from build123d import *

# Parameters (mm, degrees)
SKETCH002_W     = 160
SKETCH002_H     = 40
SKETCH002_R     = 5
PAD001_DEPTH    = 10
CHAMFER001_SIZE = 2


with BuildPart() as part:
    # Sketch002 → Pad001 (new body)
    with BuildSketch(Plane.XY):
        Rectangle(SKETCH002_W, SKETCH002_H)
        with Locations((-50, 0)):
            Circle(SKETCH002_R, mode=Mode.SUBTRACT)
        with Locations((50, 0)):
            Circle(SKETCH002_R, mode=Mode.SUBTRACT)
    extrude(amount=PAD001_DEPTH)

    # Chamfer001
    chamfer001_edges = [part.edges().sort_by_distance(p)[0] for p in [
        (-80, 0, 10),
        (0, 20, 10),
        (80, 0, 10),
        (0, -20, 10),
    ]]
    chamfer(chamfer001_edges, length=CHAMFER001_SIZE)


solid = part.part
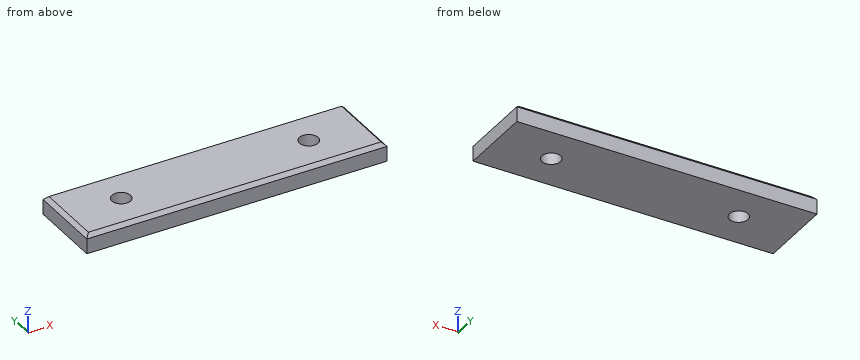
Part model, mm, in its own coordinate system. Give positions to 0.01 mm unless a question says otherwise; leave off trailing zeros. Order: outer loops, then holes, each group sorted by start corner. A loop starts at its lowest first (then second) coordinate and runs counter-clockwise, first axis right, second up. Notation, with made-up numbers: (21.5, 7.25) - (42.5, 7.25) arc R20 ccw to (42.5, 46.25) - close; hole circle Ø5 at (26, -24). An arc over 180 degrees is marked (long way). Use a Markdown table: item, result.
1) Saw through at B-B on x = 50. List the corners of the cut face in (y, z), plus the area to 3 significant figures.
Checked values:
| item | result |
|---|---|
| outline | (-20, 0) - (-5, 0) - (-5, 10) - (-18, 10) - (-20, 8) - close; (5, 0) - (20, 0) - (20, 8) - (18, 10) - (5, 10) - close |
| area | 296 mm² |
2) Saw through at C-C on z = 4.5. List the corners of the cut face in (x, y).
Checked values:
| item | result |
|---|---|
| outline | (-80, -20) - (80, -20) - (80, 20) - (-80, 20) - close; hole circle Ø10 at (-50, 0); hole circle Ø10 at (50, 0) |
3) Probe L1, parallel to Y at x = -50, z = 6; L2, parallel to X at y = -3, z = 3.25; L3, parallel to Y at x = -10.5, z = 9.75. List the from-to ranges inside material, lowest first. Write a range as from..to.
Checked values:
| item | result |
|---|---|
| L1 | -20..-5, 5..20 |
| L2 | -80..-54, -46..46, 54..80 |
| L3 | -18.25..18.25 |
4) Saw through at A-A on y = -3. List the corners of the cut face in (x, z).
Checked values:
| item | result |
|---|---|
| outline | (-80, 0) - (-54, 0) - (-54, 10) - (-78, 10) - (-80, 8) - close; (-46, 0) - (46, 0) - (46, 10) - (-46, 10) - close; (54, 0) - (80, 0) - (80, 8) - (78, 10) - (54, 10) - close |
5) Flat gauge pin, fed straight in: P1, Ø9, axis at x = -50, y = 0, coming from the +Z side. Where does the tip first touch, or does it go through?
Checked values:
| item | result |
|---|---|
| P1 | through |
